from build123d import *

# Parameters (mm, degrees)
CYLINDER_R     = 2.5
CYLINDER_DEPTH = 24
BOX_W          = 42.3
BOX_H          = 42.3
BOX_DEPTH      = 38


with BuildPart() as rotor:
    # Cylinder → Cylinder (new body)
    with BuildSketch(Plane(origin=(21.15, 21.15, 38), x_dir=(1, 0, 0), z_dir=(0, 0, 1))):
        Circle(CYLINDER_R)
    extrude(amount=CYLINDER_DEPTH)


with BuildPart() as obj1:
    # Box → Box (new body)
    with BuildSketch(Plane.XY):
        with Locations((21.15, 21.15)):
            Rectangle(BOX_W, BOX_H)
    extrude(amount=BOX_DEPTH)

    # Fusion: union Rotor
    add(rotor.part)


solid = obj1.part
Input: part model. Units: mm. Frame: model coordinates. A direction names the side the tool comes from. Give positions to 0.01 mm unless a question says otherwise; leave off trailing zeros. Order: outer loops, then holes, each group sorted by start corner. A loop starts at its lowest first (then second) coordinate and runs counter-clockwise, first axis right, second up. Notation, with made-up numbers: (40, 48) - (49, 48) arc R26 ccw to (49, 76) - close; hole circle Ø3 at (15.5, 56). An arc over 180 degrees is marked (long way). Answer as a JSON object with one key per item and string values. Group by question number.
Q1. Set-up query: faces 1 (the face through (21, 21, 0)), 2 (the face through (22.49, 23.26, 49.83)). Return all of +Z, -Z, +X, -X, +Y, -Y with unobstructed straight access to the full face (end or side cutting, diameter ignored); none if empty.
Q2. Line query: probe 1 along Z at (x, y) = (4, 31); probe 2 along X at (y, z) = (21, 44.5). Output: solid intervals per line, ascending.
Q3. Cut plane C-C, the plane x = 27.5. Output: boundary loops of the cut face in (y, z).
Q4. First-contact query: pin 1 Ø2 at (x, y) = (27, 25.5) entering from +Z. Flat tip, straight axial feed; report the tip coordinate or a pass-through.
Q5. Cut plane A-A, the plane x = 21.15. Output: boundary loops of the cut face in (y, z), then the cut area to 3 significant figures.
Results:
{
 "1": {"face 1": "-Z, +X, -X, +Y, -Y", "face 2": "+Z"},
 "2": {"probe 1": "0 to 38", "probe 2": "18.65 to 23.65"},
 "3": {"outline": "(0, 0) - (42.3, 0) - (42.3, 38) - (0, 38) - close"},
 "4": {"pin 1": "z = 38"},
 "5": {"outline": "(0, 0) - (42.3, 0) - (42.3, 38) - (23.65, 38) - (23.65, 62) - (18.65, 62) - (18.65, 38) - (0, 38) - close", "area": "1,730 mm^2"}
}
